from build123d import *

# Parameters (mm, degrees)
SKETCH_1_R                  = 200
SKETCH_1_R_2                = 150
EXTRUDE_1_DEPTH             = 15
SKETCH_2_R                  = 165
SKETCH_2_R_2                = 150
EXTRUDE_2_DEPTH             = 150
HOLE_WIZARD_M8_1_AT_2_COUNT = 2
HOLE_WIZARD_M8_1_AT_2_PITCH = 260
HOLE_WIZARD_M8_1_AT_3_COUNT = 2
HOLE_WIZARD_M8_1_AT_3_PITCH = 367.695526217
HOLE_WIZARD_M8_1_AT_4_COUNT = 2
HOLE_WIZARD_M8_1_AT_4_PITCH = 260
SKETCH_8_R                  = 75
EXTRUDE_5_DEPTH             = 165
SKETCH_11_W                 = 92.5
SKETCH_11_H                 = 102.616555874
CUT_EXTRUDE_3_DEPTH         = 27.7
SKETCH_12_W                 = 60
SKETCH_12_H                 = 102.616555874
CUT_EXTRUDE_6_DEPTH         = 8
CUT_EXTRUDE_7_DEPTH         = 220
CUT_EXTRUDE_7_DEPTH_BACK    = 165
SKETCH_14_W                 = 60
SKETCH_14_H                 = 8
SKETCH_15_R                 = 75
CUT_EXTRUDE_8_DEPTH         = 119.3
EXTRUDE_6_DEPTH             = 10


with BuildPart() as part:
    # Sketch 1 → Extrude 1 (new body)
    with BuildSketch(Plane(origin=(0, 0, 0), x_dir=(1, 0, 0), z_dir=(0, 1, 0))):
        with Locations(Location((0, 0, 0), (0, 0, 270))):
            Circle(SKETCH_1_R)
        with Locations(Location((0, 0, 0), (0, 0, 270))):
            Circle(SKETCH_1_R_2, mode=Mode.SUBTRACT)
    extrude(amount=EXTRUDE_1_DEPTH)

    # Sketch 2 → Extrude 2 (add)
    with BuildSketch(Plane(origin=(0, 15, 0), x_dir=(1, 0, 0), z_dir=(0, 1, 0))):
        with Locations(Location((0, 0, 0), (0, 0, 270))):
            Circle(SKETCH_2_R)
        with Locations(Location((0, 0, 0), (0, 0, 270))):
            Circle(SKETCH_2_R_2, mode=Mode.SUBTRACT)
    extrude(amount=EXTRUDE_2_DEPTH)

    # Sketch 5 → Hole Wizard M8 _1 (revolve, cut)
    with BuildSketch(Plane(origin=(-130, 15, -130), x_dir=(0, 0, 1), z_dir=(1, 0, 0))):
        Polygon((0, 0), (0, 15), (4.2, 15), (4.2, 9), (7.5, 9), (7.5, 0.025), (7.525, 0), align=None)
    hole_wizard_m8_1 = revolve(axis=Axis((-130, 21.35, -130), (0, -1, 0)), mode=Mode.SUBTRACT)

    # Hole Wizard M8 _1 at 2: Hole Wizard M8 _1 ×2
    with Locations(*[(i * HOLE_WIZARD_M8_1_AT_2_PITCH, 0, 0) for i in range(1, HOLE_WIZARD_M8_1_AT_2_COUNT)]):
        add(hole_wizard_m8_1, mode=Mode.SUBTRACT)

    # Hole Wizard M8 _1 at 3: Hole Wizard M8 _1 ×2
    with Locations(*[Vector(0.7071067811865476, 0, 0.7071067811865476) * (i * HOLE_WIZARD_M8_1_AT_3_PITCH) for i in range(1, HOLE_WIZARD_M8_1_AT_3_COUNT)]):
        add(hole_wizard_m8_1, mode=Mode.SUBTRACT)

    # Hole Wizard M8 _1 at 4: Hole Wizard M8 _1 ×2
    with Locations(*[(0, 0, i * HOLE_WIZARD_M8_1_AT_4_PITCH) for i in range(1, HOLE_WIZARD_M8_1_AT_4_COUNT)]):
        add(hole_wizard_m8_1, mode=Mode.SUBTRACT)


with BuildPart() as body_2:
    # Sketch 8 → Extrude 5 (new body)
    with BuildSketch(Plane.XZ):
        with Locations(Location((0, 0, 0), (0, 0, 270))):
            Circle(SKETCH_8_R)
    extrude(amount=-EXTRUDE_5_DEPTH)

    # Sketch 11 → Cut-Extrude 3 (cut)
    with BuildSketch(Plane(origin=(0, 165, 0), x_dir=(1, 0, 0), z_dir=(0, 1, 0))):
        Rectangle(SKETCH_11_W, SKETCH_11_H)
    extrude(amount=-CUT_EXTRUDE_3_DEPTH, mode=Mode.SUBTRACT)

    # Sketch 12 → Cut-Extrude 6 (cut)
    with BuildSketch(Plane(origin=(0, 137.3, 0), x_dir=(1, 0, 0), z_dir=(0, 1, 0))):
        Rectangle(SKETCH_12_W, SKETCH_12_H)
    extrude(amount=-CUT_EXTRUDE_6_DEPTH, mode=Mode.SUBTRACT)


with BuildPart() as cut_extrude_7_tool:
    # Sketch 14 → Cut-Extrude 7 (new, two sides: drawn at the far end of the back side and taken through both)
    with BuildSketch(Plane.XY.offset(-51.308277937).offset(-CUT_EXTRUDE_7_DEPTH_BACK)):
        with Locations((0, 133.3)):
            Rectangle(SKETCH_14_W, SKETCH_14_H)
    extrude(amount=CUT_EXTRUDE_7_DEPTH + CUT_EXTRUDE_7_DEPTH_BACK)


with BuildPart() as part_1:
    add(part.part)

    # Cut-Extrude 7: cut by cut_extrude_7_tool
    add(cut_extrude_7_tool.part, mode=Mode.SUBTRACT)



with BuildPart() as body_2_1:
    add(body_2.part)

    # Cut-Extrude 7: cut by cut_extrude_7_tool
    add(cut_extrude_7_tool.part, mode=Mode.SUBTRACT)

    # Sketch 15 → Cut-Extrude 8 (cut)
    with BuildSketch(Plane.XZ):
        with Locations(Location((0, 0, 0), (0, 0, 270))):
            Circle(SKETCH_15_R)
    extrude(amount=-CUT_EXTRUDE_8_DEPTH, mode=Mode.SUBTRACT)


with BuildPart() as part_2:
    add(part_1.part)

    add(body_2_1.part)  # Extrude 6 merges body 2
    # Sketch 16 → Extrude 6 (add)
    with BuildSketch(Plane.XZ.offset(-119.3)):
        with BuildLine():
            Line((-75, 129.903810568), (-75, 0))
            ThreePointArc((-75, 0), (0, 75), (75, 0))
            Line((75, 0), (75, 129.903810568))
            ThreePointArc((75, 129.903810568), (0, 150), (-75, 129.903810568))
        make_face()
    extrude(amount=-EXTRUDE_6_DEPTH)


solid = part_2.part
Here's how the part is built. I have some questions about the finished solid (model axes, mm). A direction names the side the tool comes from. Round coordinates to 2 decimals unless told otherwise and drop trailing zeros. Write each loop counter-clockwise with the first axis right and the second up, starting at its lowest first coordinate (ties: lowest second). Pieces come first, ordered by that corner, then holes.
1. For faces 1 (the flat face through (-1, 129.3, 73)), 2 (the cylindrical face through (22.528, 146.908, -71.537)), 3 (the flat face through (-75, 124, 66)), which set-ups out of +Z, -Z, +X, -X, +Y, -Y let a thin tool reach every point of the face, with its end or its side?
2. Will these pins go through, and if not, where does the flat tip stop? pin 1 Ø5 at (x, z) = (-40, -20.5) entering from +Y; pin 2 Ø3 at (x, z) = (-23.5, -24) entering from +Y; pin 3 Ø6 at (x, z) = (92.5, -122) entering from -Y; pin 4 Ø7.5 at (x, z) = (128, 129.5) entering from +Y.
3. Suppose I cut it at D-D (x = 52). List the corners of the cut face in (y, z) for me, and give its area (3 significant figures).
4. I need wall thicknesses on L1, parallel to X at y = 132.5, z = 0; L2, parallel to Z at x = 130, y = 3.95; L3, parallel to X at y = 141, z = -64. Which ranges of each line are inside material? Lowest first, please.
5. Suppose I cut it at C-C (z = 90.5). List the corners of the cut face in (x, y) for me.
6. Suppose I cut it at A-A (z = -59.5). List the corners of the cut face in (x, y) for me, and give its area (3 significant figures).
7. If we mould it in two halves opening along Y, with no side actions, what happens to faces 4 (the flat face through (0, 129.3, -156)), 5 (the cylindrical face through (134.564, 10.55, 124.048)), 6 (the flat face through (-146, 165, 36))? For each: released by +Y, released by -Y, zero draft, split by the parting line, or undercut.
8. Suppose I cut it at B-B (x = 0). State how many separate pieces and enclosed holes the cut face has, and give its area (3 significant figures).
Answer sheet:
1. face 1: none
1. face 2: +Y
1. face 3: +Y, -Y
2. pin 1: stops at y = 137.3
2. pin 2: stops at y = 129.3
2. pin 3: stops at y = 0
2. pin 4: stops at y = 6
3. outline: (0, -193.12) - (15, -193.12) - (15, -156.59) - (165, -156.59) - (165, -140.7) - (0, -140.7) - close; (0, 140.7) - (119.3, 140.7) - (119.3, -54.05) - (165, -54.05) - (165, 54.05) - (129.3, 54.05) - (129.3, 140.7) - (165, 140.7) - (165, 156.59) - (15, 156.59) - (15, 193.12) - (0, 193.12) - close
3. area: 12,100 mm2
4. L1: x = -165 to -150, -75 to -30, 30 to 75, 150 to 165
4. L2: z = -151.99 to -134.2, -125.8 to -74.83, 74.83 to 125.8, 134.2 to 151.99
4. L3: x = -152.08 to -135.66, -39.1 to 39.1, 135.66 to 152.08
5. outline: (-178.35, 0) - (-119.62, 0) - (-119.62, 165) - (-137.97, 165) - (-137.97, 15) - (-178.35, 15) - close; (-75, 119.3) - (75, 119.3) - (75, 129.3) - (-75, 129.3) - close; (119.62, 0) - (178.35, 0) - (178.35, 15) - (137.97, 15) - (137.97, 165) - (119.62, 165) - close
6. outline: (-190.94, 0) - (-137.69, 0) - (-137.69, 165) - (-153.9, 165) - (-153.9, 15) - (-190.94, 15) - close; (-45.66, 119.3) - (45.66, 119.3) - (45.66, 165) - (-45.66, 165) - close; (137.69, 0) - (190.94, 0) - (190.94, 15) - (153.9, 15) - (153.9, 165) - (137.69, 165) - close; hole (-30, 129.3) - (30, 129.3) - (30, 137.3) - (-30, 137.3) - close
6. area: 10,200 mm2
7. face 4: undercut
7. face 5: zero draft
7. face 6: released by +Y
8. separate pieces: 6
8. enclosed holes: 0
8. area: 9,320 mm2
